```python
from build123d import *

# Parameters (mm, degrees)
SKETCH1_R                      = 34.925
MAIN_BODY_DEPTH                = 63.5
SKETCH2_OUTSIDE_W              = 95.336
SKETCH2_OUTSIDE_H              = 95.336
SKETCH2_OUTSIDE_R              = 34.5
BOTTOM_STEP_DEPTH              = 5
SKETCH3_OUTSIDE_W              = 95.336
SKETCH3_OUTSIDE_H              = 95.336
SKETCH3_OUTSIDE_R              = 31.75
TOP_DIAMETER_DEPTH             = 9.52
SKETCH4_OUTSIDE_W              = 95.336
SKETCH4_OUTSIDE_H              = 95.336
SKETCH4_OUTSIDE_R              = 31.25
CUT_EXTRUDE3_DEPTH             = 1
SKETCH5_R                      = 22.5
INSERT_BORE_DEPTH              = 8
SKETCH6_R                      = 18
CUT_EXTRUDE5_DEPTH             = 64.5
SKETCH7_R                      = 21
CUT_EXTRUDE6_DEPTH             = 5
BOTTOM_EDGE_CHAMFER_SIZE2      = 0.499999887
BOTTOM_EDGE_CHAMFER_SIZE       = 0.5
TOP_FACE_CHAMFER_SIZE2         = 0.499999887
TOP_FACE_CHAMFER_SIZE          = 0.5
BODY_TO_TOP_FACE_CHAMFER_SIZE2 = 0.499999887
BODY_TO_TOP_FACE_CHAMFER_SIZE  = 0.5
SKETCH8_W                      = 1
SKETCH8_H                      = 10
SKETCH9_R                      = 3
OIL_HOLE_DEPTH                 = 35.925


with BuildPart() as part:
    # Sketch1 → Main Body (new body)
    with BuildSketch(Plane(origin=(0, 0, 0), x_dir=(1, 0, 0), z_dir=(0, 1, 0))):
        Circle(SKETCH1_R)
    extrude(amount=MAIN_BODY_DEPTH)

    # Sketch2 outside → Bottom Step (cut)
    with BuildSketch(Plane.XZ):
        Rectangle(SKETCH2_OUTSIDE_W, SKETCH2_OUTSIDE_H)
        Circle(SKETCH2_OUTSIDE_R, mode=Mode.SUBTRACT)
    extrude(amount=-BOTTOM_STEP_DEPTH, mode=Mode.SUBTRACT)

    # Sketch3 outside → Top Diameter (cut)
    with BuildSketch(Plane(origin=(0, 63.5, 0), x_dir=(1, 0, 0), z_dir=(0, 1, 0))):
        Rectangle(SKETCH3_OUTSIDE_W, SKETCH3_OUTSIDE_H)
        Circle(SKETCH3_OUTSIDE_R, mode=Mode.SUBTRACT)
    extrude(amount=-TOP_DIAMETER_DEPTH, mode=Mode.SUBTRACT)

    # Sketch4 outside → Cut-Extrude3 (cut)
    with BuildSketch(Plane(origin=(0, 53.98, 0), x_dir=(1, 0, 0), z_dir=(0, 1, 0))):
        Rectangle(SKETCH4_OUTSIDE_W, SKETCH4_OUTSIDE_H)
        Circle(SKETCH4_OUTSIDE_R, mode=Mode.SUBTRACT)
    extrude(amount=CUT_EXTRUDE3_DEPTH, mode=Mode.SUBTRACT)

    # Sketch5 → Insert Bore (cut)
    with BuildSketch(Plane(origin=(0, 63.5, 0), x_dir=(1, 0, 0), z_dir=(0, 1, 0))):
        Circle(SKETCH5_R)
    extrude(amount=-INSERT_BORE_DEPTH, mode=Mode.SUBTRACT)

    # Sketch6 → Cut-Extrude5 (cut, through all)
    with BuildSketch(Plane.XZ):
        Circle(SKETCH6_R)
    extrude(amount=-CUT_EXTRUDE5_DEPTH, mode=Mode.SUBTRACT)

    # Sketch7 → Cut-Extrude6 (cut)
    with BuildSketch(Plane.XZ):
        Circle(SKETCH7_R)
    extrude(amount=-CUT_EXTRUDE6_DEPTH, mode=Mode.SUBTRACT)

    # Bottom Edge Chamfer
    bottom_edge_chamfer_edges = [part.edges().sort_by_distance(p)[0] for p in [
        (-34.5, 0, 0),
    ]]
    chamfer(bottom_edge_chamfer_edges, length=BOTTOM_EDGE_CHAMFER_SIZE, length2=BOTTOM_EDGE_CHAMFER_SIZE2)

    # Top Face Chamfer
    top_face_chamfer_edges = [part.edges().sort_by_distance(p)[0] for p in [
        (-31.75, 63.5, 0),
    ]]
    chamfer(top_face_chamfer_edges, length=TOP_FACE_CHAMFER_SIZE, length2=TOP_FACE_CHAMFER_SIZE2)

    # Body To Top Face Chamfer
    body_to_top_face_chamfer_edges = [part.edges().sort_by_distance(p)[0] for p in [
        (-34.925, 53.98, 0),
    ]]
    chamfer(body_to_top_face_chamfer_edges, length=BODY_TO_TOP_FACE_CHAMFER_SIZE, length2=BODY_TO_TOP_FACE_CHAMFER_SIZE2)

    # Sketch8 → Oil Groove (revolve, cut)
    with BuildSketch(Plane.XY):
        with Locations((34.425, 45)):
            Rectangle(SKETCH8_W, SKETCH8_H)
    revolve(axis=Axis((0, 0, 0), (0, 1, 0)), mode=Mode.SUBTRACT)

    # Sketch9 → Oil Hole (cut, through all)
    with BuildSketch(Plane.XY):
        with Locations((0, 45)):
            Circle(SKETCH9_R)
    extrude(amount=OIL_HOLE_DEPTH, mode=Mode.SUBTRACT)


solid = part.part
```
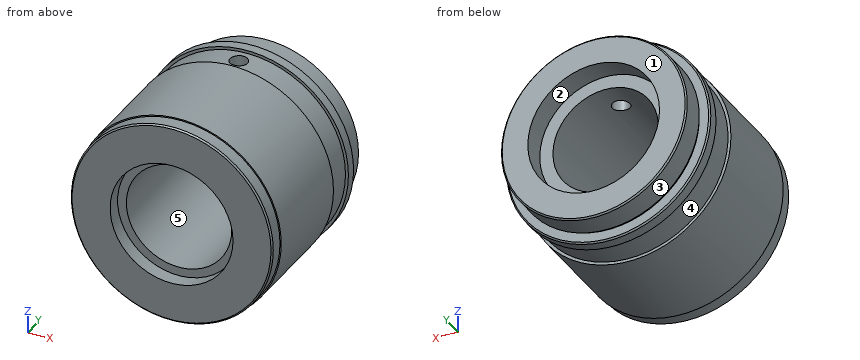
Read the model definition and answer for the solid it produces. Units are mm, in the model's axes. Face numbers are marked on the shaded views. A direction names the side the tool comes from. Coordinates: 2 decimals unless noted, no trailing zeros. Order: outer loops, then holes, each group sorted by start corner. A loop starts at its lowest first (then second) coordinate and runs counter-clockwise, first axis right, second up. Notation, with made-up numbers: (-15, 52.25) - (24, 52.25) arc R25 cw to (24, 76.25) - close; hole circle Ø5 at (-28.5, 29.5). An arc over 180 degrees is marked (long way). Answer as a JSON object with one key per item and string values. Group by question number.
Item 1: Consider probe 1 along Z at (x, y) = (0, 33) (3 decimals); probe 2 along Z at (x, y) = (0, 60). Determine where each line is inside the solid, lowest interval first. Write a range as from..to.
Item 2: The mould has two halves that part along Z. Classify the marked faces 1, 2 and 3: +Z half, -Z half, draft (parallel to the pull), parting line (faces both ways), or undercut.
Item 3: Section C-C (y = 45) is taken. Give the vertices of the cut face in (x, z) (3 decimals), plus the area to 3 significant figures.
Item 4: Section A-A (x = 0) is taken. State how many separate pieces and enclosed holes the cut face has, plus the area to 3 significant figures.
Item 5: Section B-B (y = 52.5) is taken. Give the vertices of the cut face in (x, z) (3 decimals), plus the area to 3 significant figures.
Item 6: A tool of negligible diameter and unlimited length cuts with its end or side. For the marked faces 4 and 5, from which of +Z, -Z, +X, -X, +Y, -Y can it reach the whole face along a straight path? Write none if from no direction.
Item 7: Flat-ended cylindrical pins translate along their axes: P1, Ø12, axis at y = 55, z = -25.5, coming from the -X side; P2, Ø1.5, axis at x = 26, y = 32.5, coming from the -Z side; P3, Ø4, axis at y = 28, z = -11, coming from the -X side. Find the tip coordinate at first contact, or state that the pin passes through.
Results are:
{
 "1": {"probe 1": "z = -34.925..-18, 18..34.925", "probe 2": "z = -31.75..-22.5, 22.5..31.75"},
 "2": {"face 1": "draft", "face 2": "undercut", "face 3": "parting line"},
 "3": {"outline": "(-3, 17.748) - (-3, 33.792) arc R33.925 ccw (long way) to (3, 33.792) - (3, 17.748) arc R18 cw (long way) to start", "area": "2,500 mm^2"},
 "4": {"separate pieces": "3", "enclosed holes": "0", "area": "1,870 mm^2"},
 "5": {"outline": "circle Ø69.85 at (0, 0); hole circle Ø36 at (0, 0)", "area": "2,810 mm^2"},
 "6": {"face 4": "none", "face 5": "+Y, -Y"},
 "7": {"P1": "stops at x = -28.84", "P2": "stops at z = -24.13", "P3": "stops at x = -33.75"}
}
